Can you work these out from the model? Positions are in its coordinate system, mm. Give positions to 0.01 mm unless a question says otherwise; leave off trailing zeros. Write each loop counter-clockwise with the first axis right and the second up, starting at its lowest first coordinate (ties: lowest second). Pieces come first, ordered by that corner, then holes. Notation, with made-up numbers: (87.25, 79.25) -> (131.25, 79.25) arc R11 cw to (131.25, 87.25) -> close; hole circle Ø3 at (-0.5, 35). An arc over 180 degrees is marked (long way). Answer as CSV lines item,"result". Start each with the question number.
1. If we section it at B-B on x = 11: Write out the boundary of the cut face in (y, z).
2. If we section it at D-D on x = -3: Write out the boundary of the cut face in (y, z), plus the area to 3 significant figures.
3. If we section it at A-A on z = 3.25: Write out the boundary of the cut face in (x, y).
4. I need wall thicknesses on line 1 (X direction, y = 0.5, z = 3.25); line 2 (Z direction, x = -11.5, y = 1.2); line 3 (Z direction, x = 13, y = 1.5). Which ranges of each line are inside material? Lowest first, please. Write a range as [from, to].
5. If we section it at C-C on y = 0.3: Write out the boundary of the cut face in (x, z).
```python
from build123d import *

# Parameters (mm, degrees)
RESSALTO_EXTRUS_O1_DEPTH = 2
FILETE1_R                = 1


with BuildPart() as part:
    # Esboço1 → Ressalto-extrusão1 (new body)
    with BuildSketch(Plane(origin=(0, 0, 0), x_dir=(1, 0, 0), z_dir=(0, 1, 0))):
        with BuildLine():
            ThreePointArc((0, 6), (-6.841228784, 7.123893127), (-13.763951561, 7.5))
            ThreePointArc((-13.763951561, 7.5), (-18.1422658, 7.349823523), (-22.5, 6.9))
            Line((-22.5, 6.9), (-22.5, -7.5))
            Line((-22.5, -7.5), (-2, -7.5))
            Line((-2, -7.5), (0, -5.5))
            Line((0, -5.5), (2, -7.5))
            Line((2, -7.5), (22.5, -7.5))
            Line((22.5, -7.5), (22.5, 6.9))
            ThreePointArc((22.5, 6.9), (18.1422658, 7.349823523), (13.763951559, 7.5))
            ThreePointArc((13.763951559, 7.5), (6.841228783, 7.123893127), (0, 6))
        make_face()
        with BuildLine():
            ThreePointArc((-12, 5.5), (-11, 6.5), (-10, 5.5))
            Line((-10, 5.5), (-10, -4.5))
            ThreePointArc((-10, -4.5), (-11, -5.5), (-12, -4.5))
            Line((-12, -4.5), (-12, 5.5))
        make_face(mode=Mode.SUBTRACT)
        with BuildLine():
            Line((10, -4.5), (10, 5.5))
            ThreePointArc((10, 5.5), (11, 6.5), (12, 5.5))
            Line((12, 5.5), (12, -4.5))
            ThreePointArc((12, -4.5), (11, -5.5), (10, -4.5))
        make_face(mode=Mode.SUBTRACT)
    extrude(amount=RESSALTO_EXTRUS_O1_DEPTH)

    # Filete1
    filete1_edges = [part.edges().sort_by_distance(p)[0] for p in [
        (22.5, 1, -6.9),
        (22.5, 1, 7.5),
        (2, 1, 7.5),
        (-2, 1, 7.5),
        (-22.5, 1, 7.5),
        (-22.5, 1, -6.9),
    ]]
    fillet(filete1_edges, radius=FILETE1_R)


solid = part.part
```
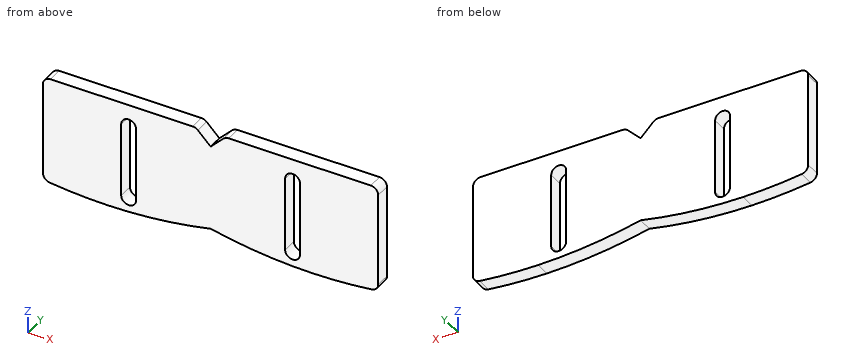
Computed values:
1,outline,"(0, -7.44) -> (2, -7.44) -> (2, -6.5) -> (0, -6.5) -> close; (0, 5.5) -> (2, 5.5) -> (2, 7.5) -> (0, 7.5) -> close"
2,outline,"(0, -6.59) -> (2, -6.59) -> (2, 7.5) -> (0, 7.5) -> close"
2,area,"28.2 mm2"
3,outline,"(-22.5, 0) -> (-12, 0) -> (-12, 2) -> (-22.5, 2) -> close; (-10, 0) -> (10, 0) -> (10, 2) -> (-10, 2) -> close; (12, 0) -> (22.5, 0) -> (22.5, 2) -> (12, 2) -> close"
4,line 1,"x = [-22.5, -12], [-10, 10], [12, 22.5]"
4,line 2,"z = [-7.46, -6.37], [5.37, 7.5]"
4,line 3,"z = [-7.5, 7.5]"
5,outline,"(-22.5, -6.02) arc R1 ccw to (-21.62, -7.01) arc R63.9 ccw to (0, -6) arc R63.9 ccw to (21.62, -7.01) arc R1 ccw to (22.5, -6.02) -> (22.5, 6.5) arc R1 ccw to (21.5, 7.5) -> (2.41, 7.5) arc R1 ccw to (1.71, 7.21) -> (0, 5.5) -> (-1.71, 7.21) arc R1 ccw to (-2.41, 7.5) -> (-21.5, 7.5) arc R1 ccw to (-22.5, 6.5) -> close; hole (-12, -5.5) arc R1 ccw to (-10, -5.5) -> (-10, 4.5) arc R1 ccw to (-12, 4.5) -> close; hole (10, -5.5) arc R1 ccw to (12, -5.5) -> (12, 4.5) arc R1 ccw to (10, 4.5) -> close"
